CAD build for the part. Positions are in the model's coordinates, mm. A direction names the side the tool comes from. Round coordinates to 2 decimals unless told otherwise and drop trailing zeros. Loops run counter-clockwise (first coordinate to the right, second up) from the corner with the lowest first, then second, coordinate; pieces in that order, holes last. Notation, with made-up numbers: M 4.25,86 L 44.25,86 A25 ccw 44.25,121 Z; hole C -25,30.25 d7. An arc over 180 degrees is marked long. Use a Markdown table: item, result. Add a question column.
(1) Flat gauge pins, fed straight in: P1, Ø3, axis at x = -24.5, y = 19, coming from the -Z side; P2, Ø5, axis at x = 16.25, y = 14, coming from the +Z side; P3, Ø10.5, axis at x = 13.5, z = -23, coming from the +Y side; P4, Ø4, axis at x = -8, y = 11, coming from the -Z side. Where does each tip first touch, or does it go through?
(2) Which spindle directions (+Z, -Z, +X, -X, +Y, -Y) get a long thin tool onto all of the face, cutting with end or side? Do faces 1 (the face through (8.25, 14.07, 0.99)), 2 (the face through (25, 13, -30.5)), 3 (the face through (21, 11, -29)). Say none if no direction does.
(3) Two-plate mould, pull along Z, no slides. Class faces 4 (the face through (-19, 1, -29)), 5 (the face through (11.4, 1, -14.3)), 6 (the face through (23, 1, -7)): released by +Z, released by -Z, zero draft, split by the parting line, or undercut.
(4) Wall check: L1, parallel to X at y = 9, z = -29.2; L2, parallel to X at y = 6.25, z = -30; L3, parallel to Y at x = 9.75, z = 0.85. Give the ranges that are in metal, low to high.
(5) Band-saw the part on B-B, the plane y = 14. Give the number of separate pieces and of enclosed holes in the cut face, and give its area (3 significant figures).
(6) Band-saw the part on A-A, the plane y = 4. Write the cut outline in (x, z).
from build123d import *

# Parameters (mm, degrees)
SKETCH_1_R          = 2
SKETCH_1_R_2        = 4
SKETCH_1_R_3        = 1.5
EXTRUDE_1_DEPTH     = 2
SKETCH_2_W          = 42
SKETCH_2_H          = 2
SKETCH_2_W_2        = 8
EXTRUDE_2_DEPTH     = 26
SKETCH_3_R          = 2
SKETCH_3_R_2        = 1.5
CUT_EXTRUDE_1_DEPTH = 51.727211632
FILLET_1_R          = 3


with BuildPart() as part:
    # 草图1 → 凸台-拉伸1 (new body)
    with BuildSketch(Plane(origin=(0, 0, 0), x_dir=(1, 0, 0), z_dir=(0, 1, 0))):
        Polygon((-29, 7), (-21, 7), (-21, 0), (21, 0), (21, 7), (29, 7), (29, 28.5), (21, 28.5), (21, 26), (19, 26), (19, 35.5), (-19, 35.5), (-19, 26), (-21, 26), (-21, 28.5), (-29, 28.5), align=None)
        with Locations(Location((-25, 12.5, 0), (0, 0, 270))):
            Circle(SKETCH_1_R, mode=Mode.SUBTRACT)
        with Locations(Location((-25, 22.5, 0), (0, 0, 270))):
            Circle(SKETCH_1_R, mode=Mode.SUBTRACT)
        with Locations(Location((25, 22.5, 0), (0, 0, 90))):
            Circle(SKETCH_1_R, mode=Mode.SUBTRACT)
        with Locations(Location((25, 12.5, 0), (0, 0, 90))):
            Circle(SKETCH_1_R, mode=Mode.SUBTRACT)
        with Locations(Location((-10.5, 22.5, 0), (0, 0, 270))):
            Circle(SKETCH_1_R_2, mode=Mode.SUBTRACT)
        with Locations(Location((-10.5, 29.5, 0), (0, 0, 270))):
            Circle(SKETCH_1_R_3, mode=Mode.SUBTRACT)
        with Locations(Location((-3.5, 22.5, 0), (0, 0, 270))):
            Circle(SKETCH_1_R_3, mode=Mode.SUBTRACT)
        with Locations(Location((-10.5, 15.5, 0), (0, 0, 270))):
            Circle(SKETCH_1_R_3, mode=Mode.SUBTRACT)
        with Locations(Location((-17.5, 22.5, 0), (0, 0, 270))):
            Circle(SKETCH_1_R_3, mode=Mode.SUBTRACT)
        with Locations(Location((3.5, 22.5, 0), (0, 0, 90))):
            Circle(SKETCH_1_R_3, mode=Mode.SUBTRACT)
        with Locations(Location((10.5, 15.5, 0), (0, 0, 90))):
            Circle(SKETCH_1_R_3, mode=Mode.SUBTRACT)
        with Locations(Location((17.5, 22.5, 0), (0, 0, 90))):
            Circle(SKETCH_1_R_3, mode=Mode.SUBTRACT)
        with Locations(Location((10.5, 22.5, 0), (0, 0, 90))):
            Circle(SKETCH_1_R_2, mode=Mode.SUBTRACT)
        with Locations(Location((10.5, 29.5, 0), (0, 0, 90))):
            Circle(SKETCH_1_R_3, mode=Mode.SUBTRACT)
        with Locations(Location((0, 12, 0), (0, 0, 270))):
            Circle(SKETCH_1_R_2, mode=Mode.SUBTRACT)
        with Locations(Location((0, 19, 0), (0, 0, 270))):
            Circle(SKETCH_1_R_3, mode=Mode.SUBTRACT)
        with Locations(Location((7, 12, 0), (0, 0, 270))):
            Circle(SKETCH_1_R_3, mode=Mode.SUBTRACT)
        with Locations(Location((0, 5, 0), (0, 0, 270))):
            Circle(SKETCH_1_R_3, mode=Mode.SUBTRACT)
        with Locations(Location((-7, 12, 0), (0, 0, 270))):
            Circle(SKETCH_1_R_3, mode=Mode.SUBTRACT)
    extrude(amount=EXTRUDE_1_DEPTH)

    # 草图2 → 凸台-拉伸2 (add)
    with BuildSketch(Plane.XZ):
        with Locations((0, 1)):
            Rectangle(SKETCH_2_W, SKETCH_2_H)
        with Locations((-25, -29.5)):
            Rectangle(SKETCH_2_W_2, SKETCH_2_H)
        with Locations((25, -29.5)):
            Rectangle(SKETCH_2_W_2, SKETCH_2_H)
    extrude(amount=-EXTRUDE_2_DEPTH)

    # 草图3 → 切除-拉伸1 (cut, through all)
    with BuildSketch(Plane.XY.offset(-30.5)):
        with Locations(Location((-24.5, 19, 0), (0, 0, 180))):
            Circle(SKETCH_3_R)
        with Locations(Location((-24.5, 9, 0), (0, 0, 180))):
            Circle(SKETCH_3_R)
        with Locations(Location((24.5, 9, 0), (0, 0, 180))):
            Circle(SKETCH_3_R)
        with Locations(Location((24.5, 19, 0), (0, 0, 180))):
            Circle(SKETCH_3_R)
        with Locations((-16.25, 14)):
            Circle(SKETCH_3_R_2)
        with Locations((-9.75, 14)):
            Circle(SKETCH_3_R_2)
        with Locations((-3.25, 14)):
            Circle(SKETCH_3_R_2)
        with Locations((3.25, 14)):
            Circle(SKETCH_3_R_2)
        with Locations((9.75, 14)):
            Circle(SKETCH_3_R_2)
        with Locations((16.25, 14)):
            Circle(SKETCH_3_R_2)
        with Locations((-9.75, 7.5)):
            Circle(SKETCH_3_R_2)
        with Locations((-9.75, 20.5)):
            Circle(SKETCH_3_R_2)
        with Locations(Location((9.75, 7.5, 0), (0, 0, 180))):
            Circle(SKETCH_3_R_2)
        with Locations(Location((9.75, 20.5, 0), (0, 0, 180))):
            Circle(SKETCH_3_R_2)
    extrude(amount=CUT_EXTRUDE_1_DEPTH, mode=Mode.SUBTRACT)

    # 圆角1
    fillet_1_edges = [part.edges().sort_by_distance(p)[0] for p in [
        (-21, 26, 1),
        (21, 26, 1),
        (-21, 26, -29.5),
        (-29, 26, -29.5),
        (29, 26, -29.5),
        (21, 26, -29.5),
        (-19, 1, -35.5),
        (19, 1, -35.5),
        (29, 1, -7),
        (-29, 1, -7),
    ]]
    fillet(fillet_1_edges, radius=FILLET_1_R)


solid = part.part
Return value:
| question | item | result |
|---|---|---|
| 1 | P1 | through |
| 1 | P2 | z = 2 |
| 1 | P3 | y = 2 |
| 1 | P4 | z = 0 |
| 2 | face 1 | +Z, -Z |
| 2 | face 2 | -Z, +X, +Y, -Y |
| 2 | face 3 | -Z, +Y, -Y |
| 3 | face 4 | zero draft |
| 3 | face 5 | undercut |
| 3 | face 6 | released by +Z |
| 4 | L1 | -29 to -26.5, -22.5 to -21, 21 to 22.5, 26.5 to 29 |
| 4 | L2 | -29 to -21, 21 to 29 |
| 4 | L3 | 0 to 6, 9 to 12.5, 15.5 to 19, 22 to 26 |
| 5 | separate pieces | 9 |
| 5 | enclosed holes | 0 |
| 5 | area | 80.0 mm^2 |
| 6 | outline | M -29,-30.5 L -21,-30.5 L -21,-28.5 L -29,-28.5 Z; M -21,0 L 21,0 L 21,2 L -21,2 Z; M 21,-30.5 L 29,-30.5 L 29,-28.5 L 21,-28.5 Z |
